Input: part model. Units: mm. Frame: model coordinates. A direction names the side the tool comes from. Coordinates: 2 decimals unless noted, no trailing zeros. Order: outer loops, then holes, each group sorted by start corner. A loop starts at its lowest first (then second) coordinate and runs counter-clockwise, first axis right, second up. Notation, with made-up numbers: (26.5, 24) -> (63.5, 24) arc R20 cw to (63.5, 63) -> close; hole circle Ø11 at (76, -39). An arc over 180 degrees is marked (long way). Write each question's results on one line, items separated by ' | '.
```python
from build123d import *

# Parameters (mm, degrees)
F1_DEPTH = 50
F3_W     = 1.5
F3_H     = 18
F4_DEPTH = 8
F6_W     = 2
F6_H     = 20
F7_DEPTH = 8


with BuildPart() as f1:
    # F0 (on Top) → F1 (new body)
    with BuildSketch(Plane.XY):
        with BuildLine():
            Line((115.8960640123, 79.0640294468), (119.7818013352, 81.7148705494))
            ThreePointArc((119.7818013352, 81.7148705494), (26.9173848976, 142.4796630761), (-81.7148705494, 119.7818013352))
            Line((-81.7148705494, 119.7818013352), (-78.783015845, 115.4841400235))
            ThreePointArc((-78.783015845, 115.4841400235), (26.1029639495, 137.6126214945), (115.8960640123, 79.0640294468))
        make_face()
    extrude(amount=F1_DEPTH)

    # F3 (on offset) → F4 (join)
    with BuildSketch(Plane(origin=(0, 0, 0), x_dir=(0.8260813885, 0.5635508314, 0), z_dir=(0.5635508314, -0.8260813885, 0))):
        with Locations((142.5461810097, 26)):
            Rectangle(F3_W, F3_H)
    extrude(amount=F4_DEPTH)

    # F6 (on offset) → F7 (cut)
    with BuildSketch(Plane(origin=(0, 0, 0), x_dir=(0.5635508314, -0.8260813885, 0), z_dir=(-0.8260813885, -0.5635508314, 0))):
        with Locations((-142.2975328202, 25)):
            Rectangle(F6_W, F6_H)
    extrude(amount=-F7_DEPTH, mode=Mode.SUBTRACT)


solid = f1.part
```
(1) Mould query, pull axis X, two halves, no side actions, for faces 6 (the face through (-76.37, 118.946, 24.86)), 7 (the face through (120.597, 77.497, 25.874)), 8 (the face through (26, 139, 0)). Classes: +X half, -X half, draft (parallel to the pull), parting line (faces both ways), or undercut.
Return value:
face 6: undercut | face 7: +X half | face 8: draft
(2) Cut plane D-D, the plane y = 93.5. Return loops of the section in (x, z).
Return value:
outline: (104.56, 0) -> (110.83, 0) -> (110.83, 50) -> (104.56, 50) -> close
(3) Pin query (flat end, axial travel): P1, Ø8, axis at y = 106.5, z = 24.5, coming from the +X side; P2, Ø1, axis at y = 133.5, z = 15, coming from the +X side; P3, Ø3, axis at x = 120.5, y = 77.5, coming from the -Z side. Return the tip coordinate at first contact, or that it passes through.
Return value:
P1: x = 102.56 | P2: x = 57.76 | P3: z = 17
(4) Reachability of faces 1 (the face through (120, 77, 17)), 2 (the face through (-77.497, 120.598, 24.86)), 3 (the face through (-80.92, 118.62, 24.65)), 4 (the face through (28.482, 142.175, 24.65)), 5 (the face through (120, 77, 35)) from +Z, -Z, +X, -X, +Y, -Y: full face, straight path, thin tool, end or side. Return the list, or none.
Return value:
face 1: -Z, +X, -Y | face 2: none | face 3: +Z, -Z, -X, -Y | face 4: +Z, -Z, +Y | face 5: +Z, +X, -Y
(5) Cut plane B-B, the plane z = 22. Return loops of the section in (x, y), plus the area to 3 significant figures.
Return value:
outline: (-81.71, 119.78) -> (-80.76, 118.38) -> (-74.15, 122.88) -> (-73.02, 121.23) -> (-79.63, 116.72) -> (-78.78, 115.48) arc R140 cw to (115.9, 79.06) -> (117.14, 79.91) -> (121.64, 73.3) -> (122.88, 74.15) -> (118.37, 80.75) -> (119.78, 81.71) arc R145 ccw to start | area: 1,100 mm2
(6) Cut plane C-C, the plane x = -47.5. Return loops of the section in (y, z).
Return value:
outline: (131.57, 0) -> (137, 0) -> (137, 50) -> (131.57, 50) -> close
(7) Cut plane A-A, the plane y = 134.5. Return loops of the section in (x, z), plus the area to 3 significant figures.
Return value:
outline: (-54.17, 0) -> (-38.5, 0) -> (-38.5, 50) -> (-54.17, 50) -> close; (39.21, 0) -> (54.17, 0) -> (54.17, 50) -> (39.21, 50) -> close | area: 1,530 mm2
(8) Line query: line 1 along X through (y, z) = (128, 32); line 2 along X through (y, z) = (129, 28); line 3 along Y through (x, z) = (37, 31.5). Output: solid intervals per line, ascending. Write a range as from..to.
Return value:
line 1: -68.12..-56.35, 57.07..68.12 | line 2: -66.21..-54.04, 54.76..66.21 | line 3: 135.12..140.2
